Read the model definition and answer for the solid it produces. Units are mm, in the model's axes. A direction names the side the tool comes from. Round coordinates to 2 decimals unless told otherwise and drop trailing zeros. Order: outer loops, then holes, each group sorted by start corner. A loop starts at its lowest first (then second) coordinate and runs counter-clockwise, first axis right, second up. Notation, with made-up numbers: (15, 88.5) -> (61, 88.5) arc R8 ccw to (61, 98.5) -> close; hole circle Ø7 at (-7, -5.75). An arc over 180 degrees is marked (long way). Use a Markdown table: item, result. Add a question column.
1. Consider L1, parallel to Z at x = -1.5, y = 1.25; L2, parallel to X at y = 3.25, z = -0.25; L3, parallel to Z at x = -2.25, y = 7.75. Determine where each line is inside the solid, lowest interval first. Write a range as [from, to].
2. For faces 4 (the face through (0, 8.4, 0.495)), 5 (the face through (-2, 6.35, -2)), determine the directions among +Z, -Z, +X, -X, +Y, -Y from which every point of the face is accessible in a straight line to the end or side of a thin tool.
3. Section A-A, the plane y = 5 is taken. Give the vertices of the cut face in (x, z).
4. Given pin 1 (1.2 mm diameter, centred on x = 1, y = 8.5, fed in from -Z); pin 2 (0.5 mm diameter, centred on x = 1.5, z = 0, fed in from +Y); pin 3 (3 mm diameter, centred on y = 7.5, z = 3, fed in from -X), each flat-ended and moving along its own axis, determine where each tip first touches the part or whether it passes through.
5. The mould has two halves that part along Z. Classify faces 1 (the face through (0, 0, 0)), 2 (the face through (0, 7.874, 0)), 3 (the face through (3.843, 6.657, 0.853)): +Z half, -Z half, draft (parallel to the pull), parting line (faces both ways), or undercut.
Autodesk Inventor part; units mm, degrees
ref_plane "YZ Plane" through (0, 0, 0) normal (1, 0, 0) x (0, 1, 0)
ref_plane "XZ Plane" through (0, 0, 0) normal (0, 1, 0) x (-1, 0, 0)
ref_plane "XY Plane" through (0, 0, 0) normal (0, 0, 1) x (1, 0, 0)
sketch "Sketch1" plane through (0, 0, 0) normal (0, 1, 0) x (-1, 0, 0)
  circle A0 centre (0, 0) radius 2.0828
  dimension "d4" = 4.1656
extrude "Body" add sketch "Sketch1" along normal blind 6.35
sketch "Sketch2" plane through (0, 0, 0) normal (1, 0, 0) x (0, 1, 0)
  line L0 (6.35, -2.0828) -> (6.35, 2.0828)
  line L1 (6.35, 0) -> (6.35, -3.7846)
  line L2 (6.8072, 0) -> (6.35, 0)
  line L3 (6.8072, 0) -> (6.8072, -3.937)
  arc A0 (6.8072, -3.937) -> (9.3815, 0) centre (5.0838, 0) ccw
  line L4 (6.5024, -3.937) -> (6.8072, -3.937)
  line L5 (6.8072, 0) -> (9.3815, 0)
  arc A1 (6.35, -3.7846) -> (6.5024, -3.937) centre (6.5024, -3.7846) ccw
  point P0 (0, 0)
  point P1 (6.35, -3.937)
  dimension "d5" = 3.937
  dimension "d13" = 0.4572
  dimension "d57" = 3.937
  dimension "d58" = 4.2977
  dimension "d59" = 0
  dimension "d67" = 0.1524
revolve "Head" add sketch "Sketch2" angle 360 about axis through (0, 6.8072, 0) along (0, -1, 0)
feature "Thread" [suppressed]
sketch "Sketch6" plane through (0, 0, 0) normal (0, 0, 1) x (1, 0, 0)
  line L0 (0, 0) -> (-1.4859, 0)
  line L1 (2.0828, 0) -> (-2.0828, 0)
  line L2 (-1.4859, 0) -> (-2.4948, 1.0089)
  line L3 (-2.4948, 1.0089) -> (-2.9651, -1.2188)
  line L4 (-2.9651, -1.2188) -> (-1.4859, -1.2188)
  line L5 (-2.0828, 0) -> (-2.0828, 6.35)
  line L6 (-1.4859, -1.2188) -> (-1.4859, 0)
  line L7 (0, -2.9358) -> (0, 9.083)
  point P0 (-2.0828, 0.5969)
  dimension "d49" = 1.4859
  dimension "d50" = 135
revolve "Tapered End" cut sketch "Sketch6" angle 360 about axis through (0, -10, 0) along (0, 1, 0)
sketch "Sketch7" plane through (0, 0, 0) normal (1, 0, 0) x (0, 1, 0)
  line L0 (31.75, 4.3688) -> (31.75, -4.3688)
  line L1 (7.874, 0.4953) -> (7.874, -0.4953)
  line L2 (7.874, 0.4953) -> (9.8806, 0.4953)
  line L3 (9.8806, 0.4953) -> (9.8806, -0.4953)
  line L4 (9.8806, -0.4953) -> (7.874, -0.4953)
  point P0 (0, 0)
  dimension "d61" = 0.9906
  dimension "d62" = 0.4953
  dimension "d65" = 7.874
  dimension "d66" = 2.0066
extrude "Flathead" cut sketch "Sketch7" against normal mid plane 12.7
sketch "Sketch5" plane through (0, 0, 0) normal (1, 0, 0) x (0, 1, 0)
  line L0 (0.0745, -1.5621) -> (-0.2261, -2.0828)
  line L1 (-0.2261, -2.0828) -> (-0.3253, -2.0828)
  line L2 (-0.3253, -2.0828) -> (-0.626, -1.5621)
  line L3 (0.0686, -2.0828) -> (-0.7252, -2.0828) construction
  line L4 (-0.626, -1.5621) -> (0.0745, -1.5621)
  line L5 (0, -1.5621) -> (31.75, -1.5621)
  point P0 (0, 0)
  dimension "d32" = 60
  dimension "a" = 0.0992
  dimension "d46" = 0.7937
  dimension "d54" = 0.0686
  dimension "d55" = 0.5207
  dimension "d56" = 0.0992
equation "\"d56\" = a"
properties part number "AScrew .250" material "VEX Aluminum Alloy 5052-H32"
Verdict:
| question | item | result |
|---|---|---|
| 1 | L1 | z = [-1.45, 1.45] |
| 1 | L2 | x = [-2.07, 2.07] |
| 1 | L3 | z = [-2.51, 2.51] |
| 2 | face 4 | +X, -X, +Y |
| 2 | face 5 | -Y |
| 3 | outline | circle Ø4.17 at (0, 0) |
| 4 | pin 1 | stops at z = -3.12 |
| 4 | pin 2 | stops at y = 7.87 |
| 4 | pin 3 | stops at x = -3.57 |
| 5 | face 1 | draft |
| 5 | face 2 | undercut |
| 5 | face 3 | parting line |
